Here's how the part is built. I have some questions about the finished solid (model axes, mm). Face numbers are marked on the shaded views. A direction names the side the tool comes from. Coordinates: 2 decimals unless noted, no trailing zeros. Write each loop counter-clockwise with the first axis right and the second up, starting at its lowest first coordinate (ties: lowest second). Pieces come first, ordered by that corner, then holes. Notation, with made-up numbers: M 26,25 L 79,25 A28 cw 79,61 Z; hole C 58,-31.5 d11. An arc over 180 degrees is marked long. Use a Markdown table: item, result.
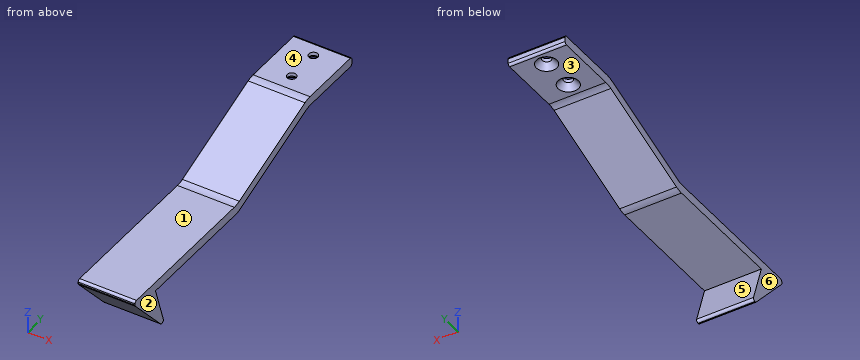
```python
from build123d import *

# Parameters (mm, degrees)
PAD_DEPTH        = 25
HOLE_D           = 4
HOLE_DEPTH       = 25
HOLE_CSINK_D     = 9
HOLE_CSINK_ANGLE = 90
FILLET_R         = 1
FILLET001_R      = 10
FILLET002_R      = 1


with BuildPart() as part:
    # Sketch001 → Pad (new body)
    with BuildSketch(Plane.YZ):
        Polygon((6, -20), (6, -18), (76.470527, -18), (125.286025, 0), (156, 0), (156, -4), (126, -4), (77.184502, -22), (20.151445, -22), (26, -40), (24, -40), align=None)
    extrude(amount=PAD_DEPTH)

    # Hole
    with Locations(Plane.YX.offset(4)):
        with Locations((134.08619, 12.5), (149.08619, 12.5)):
            CounterSinkHole(HOLE_D / 2, HOLE_CSINK_D / 2, depth=HOLE_DEPTH, counter_sink_angle=HOLE_CSINK_ANGLE)

    # Fillet
    fillet_edges = [part.edges().sort_by_distance(p)[0] for p in [
        (12.5, 6, -18),
        (12.5, 6, -20),
        (12.5, 24, -40),
        (12.5, 26, -40),
    ]]
    fillet(fillet_edges, radius=FILLET_R)

    # Fillet001
    fillet001_edges = [part.edges().sort_by_distance(p)[0] for p in [
        (12.5, 76.470527, -18),
        (12.5, 125.286025, 0),
        (12.5, 77.184502, -22),
        (12.5, 126, -4),
    ]]
    fillet(fillet001_edges, radius=FILLET001_R)

    # Fillet002
    fillet002_edges = [part.edges().sort_by_distance(p)[0] for p in [
        (12.5, 156, -4),
        (12.5, 156, 0),
    ]]
    fillet(fillet002_edges, radius=FILLET002_R)


solid = part.part
```
1. Suppose I cut it at C-C on y = 33.5. Write out the boundary of the cut face in (x, z), and give its area (3 significant figures).
Answers follow:
| item | result |
|---|---|
| outline | M 0,-22 L 25,-22 L 25,-18 L 0,-18 Z |
| area | 100 mm2 |
2. I need wall thicknesses on probe 1 along Z at (x, y) = (23.25, 133); probe 2 along Z at (x, y) = (17, 53.5); probe 3 along Y at (x, z) = (14.5, -25). Which ranges of each line are inside material? Lowest first, please.
Answers follow:
| item | result |
|---|---|
| probe 1 | z = -4 to 0 |
| probe 2 | z = -22 to -18 |
| probe 3 | y = 10.5 to 21.13 |
3. Suppose I cut it at A-A on x = 12.5. State how many separate pieces and enclosed holes the cut face has, and give its area (3 significant figures).
Answers follow:
| item | result |
|---|---|
| separate pieces | 3 |
| enclosed holes | 0 |
| area | 695 mm2 |
4. We'd pull the mould along Z, two halves only. Please class the marked faces 4, 5 and 6: +Z half, -Z half, draft (parallel to the pull), parting line (faces both ways), or undercut.
Answers follow:
| item | result |
|---|---|
| face 4 | +Z half |
| face 5 | undercut |
| face 6 | draft |
5. Suppose I cut it at B-B on x = 23.5. Write out the boundary of the cut face in (y, z).
Answers follow:
| item | result |
|---|---|
| outline | M 6,-19.62 A1 ccw 6.26,-20.29 L 23.7,-39.67 A1 ccw 24.45,-40 L 24.62,-40 A1 ccw 25.57,-38.69 L 20.15,-22 L 75.4,-22 A10 ccw 78.86,-21.38 L 124.33,-4.62 A10 cw 127.78,-4 L 155,-4 A1 ccw 156,-3 L 156,-1 A1 ccw 155,0 L 127.07,0 A10 ccw 123.61,-0.62 L 78.15,-17.38 A10 cw 74.69,-18 L 7,-18 A1 ccw 6,-19 Z |
6. Suppose I cut it at D-D on z = -9.5. Write out the boundary of the cut face in (x, y), and give its area (3 significant figures).
Answers follow:
| item | result |
|---|---|
| outline | M 0,99.52 L 25,99.52 L 25,111.08 L 0,111.08 Z |
| area | 289 mm2 |
7. Will these pins go through, and if not, where does the flat tip stop? pin 1 Ø10 at (x, z) = (13, -35) entering from -Y; pin 2 Ø1 at (x, z) = (14.5, -33) entering from +Y; pin 3 Ø10 at (x, z) = (19.5, -35) entering from +Y.
Answers follow:
| item | result |
|---|---|
| pin 1 | stops at y = 15 |
| pin 2 | stops at y = 23.89 |
| pin 3 | stops at y = 25.62 |
8. Which directions (+Z, -Z, +X, -X, +Y, -Y) give clear straight access to the entire face, cutting with the end or side of a thin tool? Please do the marked faces 1, 2 and 3.
Answers follow:
| item | result |
|---|---|
| face 1 | +Z, +X, -X, -Y |
| face 2 | +Z, -Z, +X, +Y, -Y |
| face 3 | -Z, +X, -X, +Y |
